from build123d import *

# Parameters (mm, degrees)
BOSS_EXTRUDE1_DEPTH = 45
SKETCH2_R           = 2.5
SKETCH2_R_2         = 2.25
BOSS_EXTRUDE2_DEPTH = 2


with BuildPart() as part:
    # Sketch1 → Boss-Extrude1 (new body)
    with BuildSketch(Plane.XY):
        with BuildLine():
            Line((4, 0), (21, 0))
            ThreePointArc((21, 0), (23.828427125, 1.171572875), (25, 4))
            Line((25, 4), (25, 11))
            ThreePointArc((25, 11), (23.828427125, 13.828427125), (21, 15))
            Line((21, 15), (4, 15))
            ThreePointArc((4, 15), (1.171572875, 13.828427125), (0, 11))
            Line((0, 11), (0, 4))
            ThreePointArc((0, 4), (1.171572875, 1.171572875), (4, 0))
        make_face()
    extrude(amount=BOSS_EXTRUDE1_DEPTH)

    # Sketch2 → Boss-Extrude2 (add)
    # profile 1 of 2: a face of its own
    with BuildSketch(Plane.XY.offset(45)):
        with Locations((19, 7.5)):
            Circle(SKETCH2_R)
        with Locations((19, 7.5)):
            Circle(SKETCH2_R_2, mode=Mode.SUBTRACT)
    # profile 2 of 2: a face of its own
    with BuildSketch(Plane.XY.offset(45)):
        Polygon((8.886751346, 7.5), (7.443375673, 10), (4.556624327, 10), (3.113248654, 7.5), (4.556624327, 5), (7.443375673, 5), align=None)
        Polygon((8.598076211, 7.5), (7.299038106, 9.75), (4.700961894, 9.75), (3.401923789, 7.5), (4.700961894, 5.25), (7.299038106, 5.25), align=None, mode=Mode.SUBTRACT)
    extrude(amount=BOSS_EXTRUDE2_DEPTH)


solid = part.part
Read the model definition and answer for the solid it produces. Units are mm, in the model's axes. A direction names the side the tool comes from. Coordinates: 2 decimals unless noted, no trailing zeros. Write each loop counter-clockwise with the first axis right and the second up, starting at its lowest first coordinate (ties: lowest second). Pieces come first, ordered by that corner, then holes. Notation, with made-up numbers: M 83,86.5 L 103,86.5 A23 cw 103,119.5 Z; hole C 71,18.25 d7. An arc over 180 degrees is marked long. Use a Markdown table: item, result.
Q1. Determine the mould class of faces 1 (the face through (23.859, 13.797, 22.185)), 2 (the face through (6, 9.75, 46)), 3 (the face through (21.146, 8.176, 45.986)), 4 (the face through (12, 8, 0)) for opening direction Y: released by +Y, released by -Y, zero draft, split by the parting line, or undercut.
Answer block:
| item | result |
|---|---|
| face 1 | released by +Y |
| face 2 | undercut |
| face 3 | undercut |
| face 4 | zero draft |
Q2. The part is cut by section B-B, the plane x = 19. Write down the section's boundary in (y, z).
Answer block:
| item | result |
|---|---|
| outline | M 0,0 L 15,0 L 15,45 L 10,45 L 10,47 L 9.75,47 L 9.75,45 L 5.25,45 L 5.25,47 L 5,47 L 5,45 L 0,45 Z |
Q3. Each of these flat-tipped pins is pushed along its axis until it touches: pin 1 Ø3.5 at (x, y) = (5.5, 6.5) entering from +Z; pin 2 Ø1.5 at (y, z) = (2, 38) entering from +X; pin 3 Ø1.6 at (x, z) = (6.5, 46) entering from +Y; pin 4 Ø6 at (x, y) = (22, 12.5) entering from +Z. Where does it stop, or does it pass through?
Answer block:
| item | result |
|---|---|
| pin 1 | stops at z = 47 |
| pin 2 | stops at x = 24.8 |
| pin 3 | stops at y = 10 |
| pin 4 | stops at z = 45 |
Q4. Which of the six approach directions +Z, -Z, +X, -X, +Y, -Y give full straight-line access (tool end or side, diameter ignored) to faces 5 (the face through (6, 5, 46)), 6 (the face through (6, 10, 46)), 7 (the face through (6, 5.25, 46)), 8 (the face through (3.845, 8.768, 45.986)), 9 (the face through (8.175, 8.732, 45.986))?
Answer block:
| item | result |
|---|---|
| face 5 | +Z, +X, -X, -Y |
| face 6 | +Z, +X, -X, +Y |
| face 7 | +Z |
| face 8 | +Z, -X, +Y |
| face 9 | +Z, +Y |
Q5. The part is cut by section A-A, the plane z = 22. Write down the section's boundary in (x, y).
Answer block:
| item | result |
|---|---|
| outline | M 0,4 A4 ccw 4,0 L 21,0 A4 ccw 25,4 L 25,11 A4 ccw 21,15 L 4,15 A4 ccw 0,11 Z |
Q6. The part is cut by section C-C, the plane x = 23. Write down the section's boundary in (y, z), then the cut area to 3 significant figures.
Answer block:
| item | result |
|---|---|
| outline | M 0.54,0 L 14.46,0 L 14.46,45 L 0.54,45 Z |
| area | 627 mm2 |
Q7. Straight lines are drawn through the part: L1, parallel to Y at x = 19, z = 46.5; L2, parallel to Z at x = 9, y = 6.25; L3, parallel to Y at x = 1.25, z = 30.5. For each, find the intervals that lie inside material, in ascending order. Write a range as [from, to].
Answer block:
| item | result |
|---|---|
| L1 | y = [5, 5.25], [9.75, 10] |
| L2 | z = [0, 45] |
| L3 | y = [1.1, 13.9] |
